Design review of the part built by this model. Coordinates are the model's own, in mm. Round coordinates to 2 decimals unless told otherwise and drop trailing zeros. Order: outer loops, then holes, each group sorted by start corner. A loop starts at its lowest first (then second) coordinate and runs counter-clockwise, first axis right, second up. Notation, with made-up numbers: (87.25, -29.5) - (133.25, -29.5) arc R25 cw to (133.25, 8.5) - close; hole circle Ø10 at (-20, 66). An arc over 180 degrees is marked (long way). Write item = value, one per line.
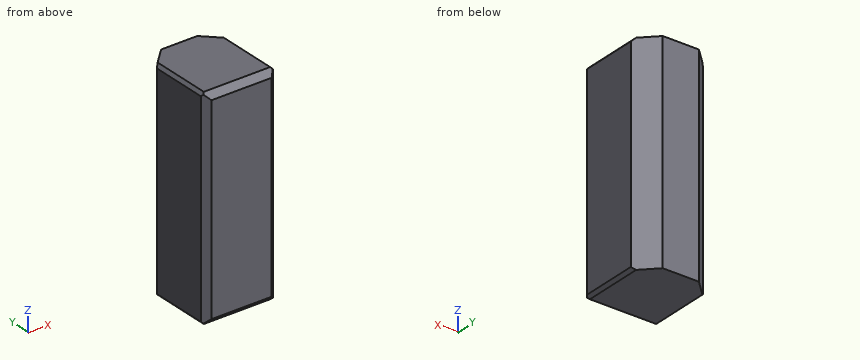
Autodesk Inventor part; units mm, degrees
ref_plane "YZ Plane" through (0, 0, 0) normal (1, 0, 0) x (0, 1, 0)
ref_plane "XZ Plane" through (0, 0, 0) normal (0, 1, 0) x (-1, 0, 0)
ref_plane "XY Plane" through (0, 0, 0) normal (0, 0, 1) x (1, 0, 0)
sketch "Sketch1" plane through (0, 0, 0) normal (0, 0, 1) x (1, 0, 0)
  line L0 (-6, 15) -> (6, 15)
  line L1 (12, 9) -> (12, -10)
  line L2 (10, -12) -> (-10, -12)
  line L3 (-12, -10) -> (-12, 9)
  line L4 (-12, 9) -> (-6, 15)
  line L5 (6, 15) -> (12, 9)
  line L6 (-12, -10) -> (-10, -12)
  line L7 (10, -12) -> (12, -10)
  point P0 (0, 0)
  point P1 (-12, 15)
  point P2 (12, -12)
  point P3 (12, 15)
  point P4 (-12, -12)
  dimension "d0" = 24
  dimension "d1" = 27
  dimension "d2" = 12
  dimension "d3" = 12
  dimension "d4" = 6
  dimension "d5" = 6
  dimension "d6" = 6
  dimension "d7" = 6
  dimension "d8" = 2
  dimension "d9" = 2
  dimension "d10" = 2
  dimension "d11" = 2
extrude "Extrusion1" add sketch "Sketch1" along normal blind 70
chamfer "Chamfer1" distance 2 angle 45 2 edges at (0, -12, 70) (0, -12, 0)
chamfer "Chamfer2" distance 1 angle 45 4 edges at (12, -0.5, 0) (-12, -0.5, 0) (-12, -0.5, 70) (12, -0.5, 70)
properties part number "battery_box"
1) We need section C-C on y = 12.5. Write out the cut boundary in (x, z).
Findings:
outline = (-8.5, 0) - (8.5, 0) - (8.5, 70) - (-8.5, 70) - close
2) We need section B-B on z = 58.5. Write out the cut boundary in (x, y).
Findings:
outline = (-12, -10) - (-10, -12) - (10, -12) - (12, -10) - (12, 9) - (6, 15) - (-6, 15) - (-12, 9) - close
3) We need section A-A on x = 7. Write out the cut boundary in (y, z), and give its area (3 significant figures).
Findings:
outline = (-12, 2) - (-10, 0) - (14, 0) - (14, 70) - (-10, 70) - (-12, 68) - close
area = 1,820 mm^2
4) To check wall thickness, follow L1, parallel to Y at x = 9, z = 6.5; L2, parallel to X at y = 10.5, z = 54; L3, parallel to X at y = 10, z = 55.5. State the ranges of each line that lie inside material, in increasing order. Write a range as from..to.
Findings:
L1 = -12..12
L2 = -10.5..10.5
L3 = -11..11
5) Clearance check with a flat-ended pin moving along its axis: pin 1 Ø1 at (x, z) = (9, 27.5) entering from +Y. State where the tip first meets the part, or that it passes through.
Findings:
pin_1 = 12.5
